Could you check a few things on this model? Use its own coordinates, in mm. Face numbers are marked on the shaded views. A direction names the side the tool comes from. Give positions to 0.01 mm unless a question says otherwise; leave off trailing zeros. Write each loop counter-clockwise with the first axis right and the second up, starting at its lowest first coordinate (ties: lowest second). Pieces come first, ordered by that corner, then holes. Notation, with made-up numbers: (52, 1) - (103, 1) arc R22 ccw to (103, 35) - close; hole circle Ø9 at (-21, 67.25). An arc over 180 degrees is marked (long way). Answer in a Markdown table with one row per item.
from build123d import *

# Parameters (mm, degrees)
SKETCH1_W                = 44.25
SKETCH1_H                = 19.9
SKETCH1_R                = 1
BOSS_EXTRUDE1_DEPTH      = 1
SKETCH2_W                = 7.4
SKETCH2_H                = 15
BOSS_EXTRUDE2_DEPTH      = 5.7
SKETCH3_W                = 13.6
SKETCH3_H                = 4.3
CUT_EXTRUDE1_DEPTH       = 6
SKETCH4_W                = 11.2
SKETCH4_H                = 5
BOSS_EXTRUDE3_DEPTH      = 5
SKETCH5_R                = 1.25
CUT_EXTRUDE2_DEPTH       = 8
BOSS_EXTRUDE4_DEPTH      = 0.5
BOSS_EXTRUDE4_DEPTH_BACK = 5.7


with BuildPart() as part:
    # Sketch1 → Boss-Extrude1 (new body)
    with BuildSketch(Plane(origin=(0, 0, 0), x_dir=(1, 0, 0), z_dir=(0, 1, 0))):
        Rectangle(SKETCH1_W, SKETCH1_H)
        with Locations(Location((-7.625, 6.8, 0), (0, 0, 270))):
            Circle(SKETCH1_R, mode=Mode.SUBTRACT)
        with Locations(Location((-7.625, -6.8, 0), (0, 0, 270))):
            Circle(SKETCH1_R, mode=Mode.SUBTRACT)
    extrude(amount=BOSS_EXTRUDE1_DEPTH)

    # Sketch2 → Boss-Extrude2 (add)
    with BuildSketch(Plane(origin=(0, 1, 0), x_dir=(1, 0, 0), z_dir=(0, 1, 0))):
        with Locations((-21.625, 0)):
            Rectangle(SKETCH2_W, SKETCH2_H)
    extrude(amount=BOSS_EXTRUDE2_DEPTH)

    # Sketch3 → Cut-Extrude1 (cut)
    with BuildSketch(Plane.ZY.offset(25.325)):
        with Locations((0, 3.85)):
            Rectangle(SKETCH3_W, SKETCH3_H)
    extrude(amount=-CUT_EXTRUDE1_DEPTH, mode=Mode.SUBTRACT)

    # Sketch4 → Boss-Extrude3 (add)
    with BuildSketch(Plane(origin=(0, 1, 0), x_dir=(1, 0, 0), z_dir=(0, 1, 0))):
        with Locations((17.025, -6.45)):
            Rectangle(SKETCH4_W, SKETCH4_H)
    extrude(amount=BOSS_EXTRUDE3_DEPTH)

    # Sketch5 → Cut-Extrude2 (cut)
    with BuildSketch(Plane(origin=(22.625, 0, 0), x_dir=(0, 0, -1), z_dir=(1, 0, 0))):
        with Locations((-6.45, 4)):
            Circle(SKETCH5_R)
    extrude(amount=-CUT_EXTRUDE2_DEPTH, mode=Mode.SUBTRACT)

    # Sketch6 → Boss-Extrude4 (add, two sides: drawn at the far end of the back side and taken through both)
    with BuildSketch(Plane(origin=(22.125, 0, 0), x_dir=(0, 0, -1), z_dir=(1, 0, 0)).offset(-BOSS_EXTRUDE4_DEPTH_BACK)):
        with BuildLine():
            Line((3.879166952, 1), (7.879166952, 1))
            Line((7.879166952, 1), (8.751177801, 1.906891284))
            ThreePointArc((8.751177801, 1.906891284), (8.950428623, 2.991721383), (8.030344737, 3.6))
            Line((8.030344737, 3.6), (3.727989167, 3.6))
            ThreePointArc((3.727989167, 3.6), (2.80790528, 2.991721383), (3.007156102, 1.906891284))
            Line((3.007156102, 1.906891284), (3.879166952, 1))
        make_face()
        with BuildLine():
            Line((3.985603275, 1.25), (7.772730629, 1.25))
            Line((7.772730629, 1.25), (8.570969535, 2.080168463))
            ThreePointArc((8.570969535, 2.080168463), (8.720407651, 2.893791037), (8.030344737, 3.35))
            Line((8.030344737, 3.35), (3.727989167, 3.35))
            ThreePointArc((3.727989167, 3.35), (3.037926252, 2.893791037), (3.187364368, 2.080168463))
            Line((3.187364368, 2.080168463), (3.985603275, 1.25))
        make_face(mode=Mode.SUBTRACT)
    extrude(amount=BOSS_EXTRUDE4_DEPTH + BOSS_EXTRUDE4_DEPTH_BACK)


solid = part.part
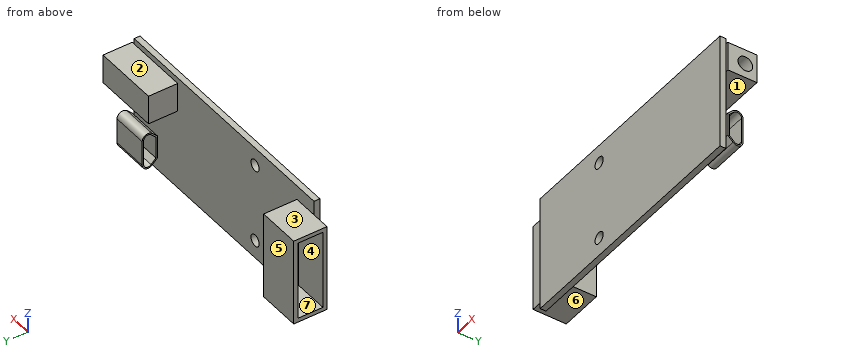
1) We'd pull the mould along Z, two halves only. Please class the marked faces 4, 5, 6 and 7: +Z half, -Z half, draft (parallel to the pull), parting line (faces both ways), or undercut.
Check values:
| item | result |
|---|---|
| face 4 | undercut |
| face 5 | draft |
| face 6 | -Z half |
| face 7 | undercut |
2) On a 3-axis mill with a long thin cutter (end or side, diameter ignored), from which of +Z, -Z, +X, -X, +Y, -Y can I reach the whole of each face in a straight line? I mean the marked faces 1, 2 and 3. Say none if no direction works.
Check values:
| item | result |
|---|---|
| face 1 | +X, +Y |
| face 2 | +Z, +X, -X, +Y |
| face 3 | +Z, -X, +Y |
3) If I drill on line 1 (X direction, y = 2.25, z = 4.75) (3 decimals); line 2 (Y direction, x = 19.25, z = 6.45); line 3 (X direction, y = 0.7, z = 6.8) (3 decimals), over which ranges is the centre line in solid material (lowest first)?
Check values:
| item | result |
|---|---|
| line 1 | x = -19.325 to -17.925, 11.425 to 22.625 |
| line 2 | y = 0 to 2.75, 5.25 to 6 |
| line 3 | x = -22.125 to -8.625, -6.625 to 22.125 |
4) Imagine slicing it at C-C (x = -18.5). List the corners of the cut face in (y, z) for me, then the cut area to 3 significant figures.
Check values:
| item | result |
|---|---|
| outline | (0, -9.95) - (1, -9.95) - (1, -7.5) - (6.7, -7.5) - (6.7, 7.5) - (1, 7.5) - (1, 9.95) - (0, 9.95) - close |
| area | 105 mm2 |
5) Will these pins go through, and if not, where does the flat tip stop? P1, Ø1.3, axis at x = 20.5, z = -6, coming from the +Y side; P2, Ø3, axis at x = -7.625, z = -6.8, coming from the +Y side; P3, Ø1.1, axis at y = 0.5, z = -3.5, coming from the +X side (3 decimals).
Check values:
| item | result |
|---|---|
| P1 | stops at y = 3.6 |
| P2 | stops at y = 1 |
| P3 | stops at x = 22.125 |
6) Imagine slicing it at B-B (z = 8.25). List the corners of the cut face in (x, y) for me (3 decimals).
Check values:
| item | result |
|---|---|
| outline | (-22.125, 0) - (22.125, 0) - (22.125, 1) - (22.625, 1) - (22.625, 6) - (11.425, 6) - (11.425, 1) - (-22.125, 1) - close |
7) Imagine slicing it at A-A (x = 15.5). List the corners of the cut face in (y, z) for me, then the cut area to 3 significant figures.
Check values:
| item | result |
|---|---|
| outline | (0, -9.95) - (1, -9.95) - (1, 3.95) - (6, 3.95) - (6, 8.95) - (1, 8.95) - (1, 9.95) - (0, 9.95) - close; hole circle Ø2.5 at (4, 6.45) |
| area | 40.0 mm2 |
8) Imagine slicing it at D-D (x = 5.5). List the corners of the cut face in (y, z) for me, then the cut area to 3 significant figures.
Check values:
| item | result |
|---|---|
| outline | (0, -9.95) - (1, -9.95) - (1, 9.95) - (0, 9.95) - close |
| area | 19.9 mm2 |
